Verification items for the finished model (mm, model axes). Round coordinates to 2 decimals unless told otherwise and drop trailing zeros. Loops run counter-clockwise (first coordinate to the right, second up) from the corner with the lowest first, then second, coordinate; pieces in that order, holes last. Notation, with made-up numbers: (74.5, -38) -> (87.5, -38) arc R8 ccw to (87.5, -29) -> close; hole circle Ø3 at (-7, 56.5). An arc over 180 degrees is marked (long way). Use a Markdown table: item, result. Add a question column.
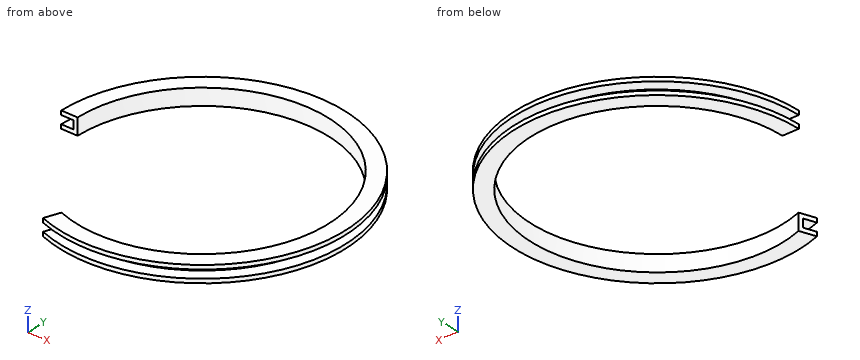
Autodesk Inventor part; units mm, degrees
ref_plane "YZ Plane" through (0, 0, 0) normal (1, 0, 0) x (0, 1, 0)
ref_plane "XZ Plane" through (0, 0, 0) normal (0, 1, 0) x (-1, 0, 0)
ref_plane "XY Plane" through (0, 0, 0) normal (0, 0, 1) x (1, 0, 0)
sketch "Sketch1" plane through (0, 0, 0) normal (0, 1, 0) x (-1, 0, 0)
  line L0 (0, 0) -> (0, 6.35)
  line L1 (0, 6.35) -> (12.7, 6.35)
  line L2 (12.7, 6.35) -> (12.7, 3.175)
  line L3 (12.7, 3.175) -> (3.175, 3.175)
  line L4 (15.24, 0) -> (-2.54, 0) construction
  line L5 (3.175, 3.175) -> (3.175, 0)
  line L6 (0, 0) -> (0, -6.35)
  line L7 (0, -6.35) -> (12.7, -6.35)
  line L8 (12.7, -6.35) -> (12.7, -3.175)
  line L9 (12.7, -3.175) -> (3.175, -3.175)
  line L10 (3.175, -3.175) -> (3.175, 0)
  dimension "d0" = 6.35
  dimension "d1" = 3.175
  dimension "d2" = 12.7
  dimension "d3" = 3.175
sketch "Sketch2" plane through (0, 0, 0) normal (0, 0, 1) x (1, 0, 0)
  line L0 (-75.0085, 0) -> (283.7112, 0)
  arc A0 (63.926, -91.2958) -> (0, 0) centre (97.155, 0) ccw
  line L1 (97.155, 0) -> (63.926, -91.2958) construction
  dimension "d4" = 194.31
  dimension "d6" = 70
sweep "Sweep1" add profiles "Sketch1" path "Sketch2" path curves A0
properties part number "3510K4"
1) Sectioned sample at B-B on y = 82.5. Enter the section's corners in (x, z) (3 decimals), then the cut area to 3 significant figures.
2) Sectioned sample at D-D on y = -88. Enter the section's corners in (x, z) (3 decimals), then the cut area to 3 significant figures.
3) Sectioned sample at A-A on x = 186. Enter the section's corners in (y, z) (3 decimals), then the cut area to 3 significant figures.
4) Sectioned sample at C-C on x = 36.5. Enter the section's corners in (y, z) (3 decimals), then the cut area to 3 significant figures.
5) Go/stop test with flat-tipped pins: pin 1 (6.5 mm diameter, centred on x = -9.5, z = 1.5, fed in from -Y); pin 2 (3 mm diameter, centred on x = 22.5, z = -1.5, fed in from -Y); pin 3 (6 mm diameter, centred on y = -87, z = 1.5, fed in from -X). Record where each tip stops, or that it passes through.
6) Thickness scan on line 1 (X direction, y = 52.5, z = -4); line 2 (Y direction, x = 68.5, z = 5); line 3 (Y direction, x = 134, z = 1.75). Record the ranges inside material, lowest first.
Geometry results:
| question | item | result |
|---|---|---|
| 1 | outline | (24.616, -6.35) -> (45.844, -6.35) -> (45.844, 6.35) -> (24.616, 6.35) -> (24.616, 3.175) -> (40.06, 3.175) -> (40.06, -3.175) -> (24.616, -3.175) -> close; (148.466, -6.35) -> (169.694, -6.35) -> (169.694, -3.175) -> (154.25, -3.175) -> (154.25, 3.175) -> (169.694, 3.175) -> (169.694, 6.35) -> (148.466, 6.35) -> close |
| 1 | area | 343 mm^2 |
| 2 | outline | (138.326, -6.35) -> (162.913, -6.35) -> (162.913, -3.175) -> (145.343, -3.175) -> (145.343, 3.175) -> (162.913, 3.175) -> (162.913, 6.35) -> (138.326, 6.35) -> close |
| 2 | area | 201 mm^2 |
| 3 | outline | (-64.612, -6.35) -> (-39.315, -6.35) -> (-39.315, 6.35) -> (-64.612, 6.35) -> (-64.612, 3.175) -> (-46.612, 3.175) -> (-46.612, -3.175) -> (-64.612, -3.175) -> close; (39.315, -6.35) -> (64.612, -6.35) -> (64.612, -3.175) -> (46.612, -3.175) -> (46.612, 3.175) -> (64.612, 3.175) -> (64.612, 6.35) -> (39.315, 6.35) -> close |
| 3 | area | 414 mm^2 |
| 4 | outline | (75.895, -6.35) -> (91.592, -6.35) -> (91.592, -3.175) -> (79.919, -3.175) -> (79.919, 3.175) -> (91.592, 3.175) -> (91.592, 6.35) -> (75.895, 6.35) -> close |
| 4 | area | 125 mm^2 |
| 5 | pin 1 | y = 0 |
| 5 | pin 2 | y = 60.33 |
| 5 | pin 3 | x = 133.75 |
| 6 | line 1 | 0.66 to 15.41, 178.9 to 193.65 |
| 6 | line 2 | -106.05 to -92.83, 92.83 to 106.05 |
| 6 | line 3 | -93.32 to -89.9, 89.9 to 93.32 |
